Check sheet for the modelled part. Datum: model origin and axes. Units: mm. Face numbers are marked on the shaded views. Round coordinates to 2 decimals unless told otherwise and drop trailing zeros. Write each loop counter-clockwise with the first axis right and the second up, starting at its lowest first coordinate (ties: lowest second). Pieces come first, ordered by that corner, then holes. Notation, with made-up numbers: (34.5, -16) -> (78.5, -16) arc R17 ccw to (78.5, 2) -> close; hole circle Ø9 at (42, 76). An arc over 180 degrees is marked (long way). One line per item, written item: value.
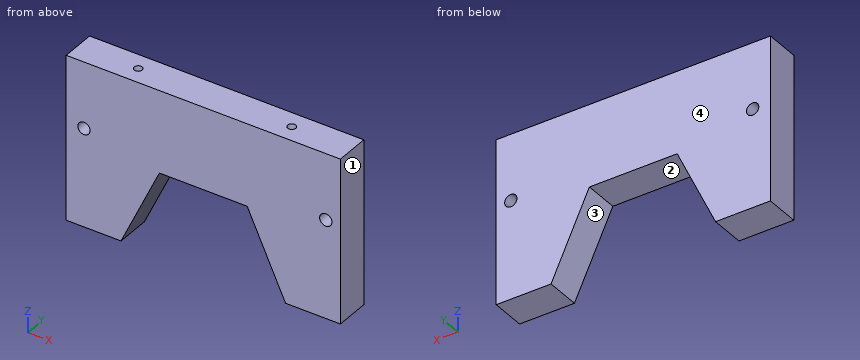
from build123d import *

# Parameters (mm, degrees)
BOSS_EXTRUDE1_DEPTH = 12.6
SKETCH2_R           = 1.5
CUT_EXTRUDE1_DEPTH  = 20
CUT_EXTRUDE2_REACH  = 14.6
SKETCH3_R           = 2.25


with BuildPart() as part:
    # Sketch1 → Boss-Extrude1 (new body)
    with BuildSketch(Plane(origin=(0, 0, 0), x_dir=(1, 0, 0), z_dir=(0, 1, 0))):
        Polygon((-30, 30), (-16.00813249, 0), (16.00813249, 0), (30, 30), (50, 30), (50, -30), (-50, -30), (-50, 30), align=None)
    extrude(amount=BOSS_EXTRUDE1_DEPTH)

    # Sketch2 → Cut-Extrude1 (cut)
    with BuildSketch(Plane.XY.offset(30)):
        with Locations((-28, 6.3)):
            Circle(SKETCH2_R)
        with Locations((28, 6.3)):
            Circle(SKETCH2_R)
    extrude(amount=-CUT_EXTRUDE1_DEPTH, mode=Mode.SUBTRACT)

    # Sketch3 → Cut-Extrude2 (cut, up to next)
    with BuildSketch(Plane.XZ, mode=Mode.PRIVATE) as cut_extrude2_sk1:
        with Locations((44.671841303, 5.85113754)):
            Circle(SKETCH3_R)
    cut_extrude2_tool1 = extrude(cut_extrude2_sk1.sketch, amount=-CUT_EXTRUDE2_REACH, mode=Mode.PRIVATE) & part.part
    add(cut_extrude2_tool1.solids().sort_by_distance((44.671841, 0, 5.851138))[0], mode=Mode.SUBTRACT)
    # Sketch3 → Cut-Extrude2 (cut, up to next)
    with BuildSketch(Plane.XZ, mode=Mode.PRIVATE) as cut_extrude2_sk2:
        with Locations((-43.519626776, 5.85113754)):
            Circle(SKETCH3_R)
    cut_extrude2_tool2 = extrude(cut_extrude2_sk2.sketch, amount=-CUT_EXTRUDE2_REACH, mode=Mode.PRIVATE) & part.part
    add(cut_extrude2_tool2.solids().sort_by_distance((-43.519627, 0, 5.851138))[0], mode=Mode.SUBTRACT)


solid = part.part
Item 1: Depth check by flat-ended pin: pin 1 (0.9 mm diameter, centred on x = 28, y = 6, fed in from +Z); pin 2 (3.5 mm diameter, centred on x = 28, y = 6.3, fed in from -Z); pin 3 (6.5 mm diameter, centred on x = 3.5, y = 7.5, fed in from -Z). Enter the tip coordinate at first touch or a pass-through.
Result set:
pin 1: z = 10
pin 2: z = -29.46
pin 3: z = 0
Item 2: Release check for a two-part mould opening along X. For the marked faces 1, 2, 3 and 4 record: pulls with the +X half, pulls with the -X half, needs draft (parallel to the pull), parting line crosses it, or undercut.
Result set:
face 1: pulls with the +X half
face 2: undercut
face 3: undercut
face 4: needs draft
Item 3: Sectioned sample at D-D (y = 6.3). Enter the section's corners in (x, z).
Result set:
outline: (-50, -30) -> (-30, -30) -> (-16.01, 0) -> (16.01, 0) -> (30, -30) -> (50, -30) -> (50, 30) -> (29.5, 30) -> (29.5, 10) -> (26.5, 10) -> (26.5, 30) -> (-26.5, 30) -> (-26.5, 10) -> (-29.5, 10) -> (-29.5, 30) -> (-50, 30) -> close; hole circle Ø4.5 at (-43.52, 5.85); hole circle Ø4.5 at (44.67, 5.85)
Item 4: Sectioned sample at B-B (x = -43). Enter the section's corners in (y, z).
Result set:
outline: (0, -30) -> (12.6, -30) -> (12.6, 3.66) -> (0, 3.66) -> close; (0, 8.04) -> (12.6, 8.04) -> (12.6, 30) -> (0, 30) -> close
Item 5: Material ranges on line 1 along X through (y, z) = (6.75, -14.5); line 2 along Z through (x, y) = (15.5, 8.5); line 3 along X through (y, z) = (1, -5), recorded low to high.
Result set:
line 1: -50 to -22.77, 22.77 to 50
line 2: 0 to 30
line 3: -50 to -18.34, 18.34 to 50
Item 6: Sectioned sample at A-A (z = -13.5). Enter the section's corners in (x, y).
Result set:
outline: (-50, 0) -> (-22.3, 0) -> (-22.3, 12.6) -> (-50, 12.6) -> close; (22.3, 0) -> (50, 0) -> (50, 12.6) -> (22.3, 12.6) -> close
Item 7: Sectioned sample at C-C (z = 7). Enter the section's corners in (x, y), then the cut area to 3 significant figures.
Result set:
outline: (-50, 0) -> (-45.45, 0) -> (-45.45, 12.6) -> (-50, 12.6) -> close; (-41.59, 0) -> (42.74, 0) -> (42.74, 12.6) -> (-41.59, 12.6) -> close; (46.61, 0) -> (50, 0) -> (50, 12.6) -> (46.61, 12.6) -> close
area: 1,160 mm^2
